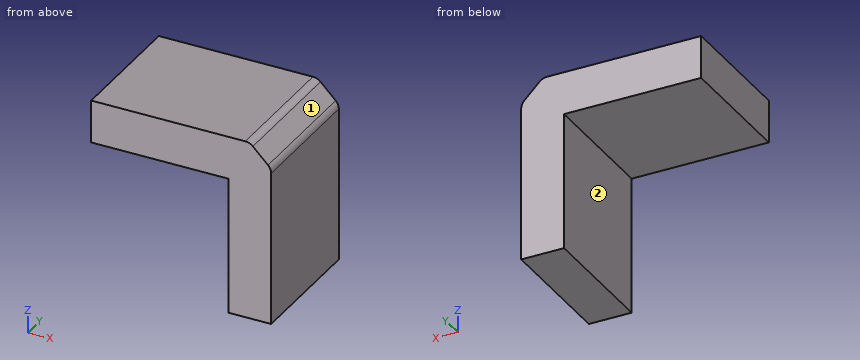
```python
from build123d import *

# Parameters (mm, degrees)
BOSS_EXTRUDE1_DEPTH = 60
CHAMFER1_SIZE       = 10
FILLET1_R           = 5


with BuildPart() as part:
    # Sketch1 → Boss-Extrude1 (new body)
    with BuildSketch(Plane(origin=(0, 0, 0), x_dir=(1, 0, 0), z_dir=(0, 1, 0))):
        Polygon((22, 42), (22, -22), (-42, -22), (-42, -42), (42, -42), (42, 42), align=None)
    extrude(amount=BOSS_EXTRUDE1_DEPTH)

    # Chamfer1
    chamfer1_edges = [part.edges().sort_by_distance(p)[0] for p in [
        (42, 30, 42),
    ]]
    chamfer(chamfer1_edges, length=CHAMFER1_SIZE)

    # Fillet1
    fillet1_edges = [part.edges().sort_by_distance(p)[0] for p in [
        (42, 30, 32),
        (32, 30, 42),
    ]]
    fillet(fillet1_edges, radius=FILLET1_R)


solid = part.part
```
Model file for the job. Use its own axes, mm. Face numbers are marked on the shaded views. A direction names the side the tool comes from. Round coordinates to 2 decimals unless told otherwise and drop trailing zeros. Order: outer loops, then holes, each group sorted by start corner. A loop starts at its lowest first (then second) coordinate and runs counter-clockwise, first axis right, second up. Notation, with made-up numbers: M 12.25,0 L 45.25,0 A14 cw 45.25,8 Z; hole C -27,4.25 d8. An arc over 180 degrees is marked long. Use CSV: the item, a comma, the result in double quotes.
Item 1: Saw through at A-A (y = 21.5). List the corners of the cut face in (x, z).
Worked answers:
outline,"M -42,22 L 22,22 L 22,-42 L 42,-42 L 42,29.93 A5 ccw 40.54,33.46 L 33.46,40.54 A5 ccw 29.93,42 L -42,42 Z"
Item 2: Saw through at C-C (x = -27). List the corners of the cut face in (y, z), plus the area to 3 significant figures.
Worked answers:
outline,"M 0,22 L 60,22 L 60,42 L 0,42 Z"
area,"1,200 mm²"
Item 3: Probe probe 1 along X at (y, z) = (36.5, -34); probe 2 along Z at (x, y) = (38.5, 8). List the from-to ranges inside material, lowest first.
Worked answers:
probe 1,"22 to 42"
probe 2,"-42 to 35.5"
Item 4: Pin check, flat tips, straight feed: pin 1 (8 mm diameter, centred on y = 40, z = -22, fed in from -X); pin 2 (12 mm diameter, centred on x = 1.5, y = 41.5, fed in from -Z). Stop position of each tip, or through.
Worked answers:
pin 1,"x = 22"
pin 2,"z = 22"
Item 5: Saw through at B-B (z = 35). List the corners of the cut face in (x, y), plus the area to 3 significant figures.
Worked answers:
outline,"M -42,0 L 39,0 L 39,60 L -42,60 Z"
area,"4,860 mm²"
Item 6: Which spindle directions (+Z, -Z, +X, -X, +Y, -Y) get a long thin tool onto all of the face, cutting with end or side? Do the marked faces 1 and 2. Say none if no direction does.
Worked answers:
face 1,"+Z, +X, +Y, -Y"
face 2,"-Z, -X, +Y, -Y"
